CAD build for the part. Positions are in the model's coordinates, mm. A direction names the side the tool comes from. Coordinates: 2 decimals unless noted, no trailing zeros. Loops run counter-clockwise (first coordinate to the right, second up) from the corner with the lowest first, then second, coordinate; pieces in that order, holes last. Notation, with made-up numbers: (-29.5, -2) -> (-5.5, -2) arc R33 cw to (-5.5, 29) -> close; hole circle Ø7 at (32, 31.5). An arc over 180 degrees is marked (long way). Write item = value, one per line. Start each with the question number.
(1) Band-saw the part on C-C (z = 0). Write the cut outline in (x, y), and give its area (3 significant figures).
(2) Tool access for faces 1 (the face through (4.6, 80, 23)), 2 (the face through (0, 80, 20.945)), 3 (the face through (-4.6, 80, 23)), 4 (the face through (-0.06, 80.01, 25.96)): list every direction of +Z, -Z, +X, -X, +Y, -Y with a clear straight run to the whole face (end or side of a thin tool).
(3) Band-saw the part on A-A (x = 0). Write the cut outline in (y, z) (3 decimals), and give its area (3 significant figures).
(4) Band-saw the part on B-B (y = 109.5). Write the cut outline in (x, z) (3 decimals), and give its area (3 significant figures).
(5) Drill centre lines: line 1 (Y direction, x = 54, z = -30.5); line 2 (X direction, y = 123.5, z = 23.5); line 3 (X direction, y = 9.5, z = -66). Where is each one in solid material? Low to high. Write a range as from..to.
(6) Flat gauge pins, fed straight in: P1, Ø8, axis at x = 4, y = 24, coming from the +Z side; P2, Ø5, axis at x = -26, z = 62, coming from the +Y side; P3, Ø10, axis at y = 28, z = 17, coming from the +X side; P4, Ø4, axis at x = 17, z = -60, coming from the -Y side. Where does each tip first touch, or does it go through?
```python
from build123d import *

# Parameters (mm, degrees)
SKETCH1_R           = 88.009986391
BOSS_EXTRUDE1_DEPTH = 10
BOSS_EXTRUDE5_DEPTH = 142


with BuildPart() as part:
    # Sketch1 → Boss-Extrude1 (new body)
    with BuildSketch(Plane(origin=(0, 0, 0), x_dir=(1, 0, 0), z_dir=(0, 1, 0))):
        with Locations(Location((0, 0, 0), (0, 0, 270))):
            Circle(SKETCH1_R)
    extrude(amount=BOSS_EXTRUDE1_DEPTH)

    # Sketch3 → Boss-Extrude5 (add)
    with BuildSketch(Plane(origin=(0, 10, 0), x_dir=(1, 0, 0), z_dir=(0, 1, 0))):
        with BuildLine():
            Line((-4.6, -20.945), (-4.6, -25.549199596))
            ThreePointArc((-4.6, -25.549199596), (0, -25.96), (4.6, -25.549199596))
            Line((4.6, -25.549199596), (4.6, -20.945))
            Line((4.6, -20.945), (-4.6, -20.945))
        make_face()
    extrude(amount=BOSS_EXTRUDE5_DEPTH)


solid = part.part
```
Findings below:
q1.outline = (-88.01, 0) -> (88.01, 0) -> (88.01, 10) -> (-88.01, 10) -> close
q1.area = 1,760 mm²
q2.face_1 = +Z, -Z, +X, +Y
q2.face_2 = -Z, +X, -X, +Y
q2.face_3 = +Z, -Z, -X, +Y
q2.face_4 = +Z, +Y
q3.outline = (0, -88.01) -> (10, -88.01) -> (10, 20.945) -> (152, 20.945) -> (152, 25.96) -> (10, 25.96) -> (10, 88.01) -> (0, 88.01) -> close
q3.area = 2,470 mm²
q4.outline = (-4.6, 20.945) -> (4.6, 20.945) -> (4.6, 25.549) arc R25.96 ccw to (-4.6, 25.549) -> close
q4.area = 44.9 mm²
q5.line_1 = 0..10
q5.line_2 = -4.6..4.6
q5.line_3 = -58.22..58.22
q6.P1 = 25.96
q6.P2 = 10
q6.P3 = 4.6
q6.P4 = 0
